```python
from build123d import *

# Parameters (mm, degrees)
SKETCH_1_W           = 23.4
SKETCH_1_H           = 23.4
EXTRUDE_1_DEPTH      = 38
CUT_EXTRUDE_START    = -4.6
SKETCH_1_3_W         = 20.4
SKETCH_1_3_H         = 17
CUT_EXTRUDE_1_DEPTH  = 37.846109588
CUT_EXTRUDE_START_2  = -1
SKETCH_1_4_W         = 10.2
SKETCH_1_4_H         = 10.2
CUT_EXTRUDE_2_DEPTH  = 41.446109588
CHAMFER_2_SIZE       = 3
CUT_EXTRUDE_3_DEPTH  = 47.135127614
CUT_EXTRUDE_4_REACH  = 46.688
CUT_EXTRUDE_5_DEPTH  = 43.900466198
CUT_EXTRUDE_6_DEPTH  = 42.340657953
SKETCH_10_W          = 4
SKETCH_10_H          = 1
CUT_EXTRUDE_10_DEPTH = 12
HOLE_WIZARD_1_D      = 1.8
HOLE_WIZARD_1_DEPTH  = 3.6


with BuildPart() as part:
    # 草图1 → 凸台-拉伸1 (new body)
    with BuildSketch(Plane.XY):
        Rectangle(SKETCH_1_W, SKETCH_1_H)
    extrude(amount=-EXTRUDE_1_DEPTH)

    # 草图1<3> → 切除-拉伸1 (cut, through all)
    with BuildSketch(Plane.XY.offset(CUT_EXTRUDE_START)):
        with Locations((0, 0.8)):
            Rectangle(SKETCH_1_3_W, SKETCH_1_3_H)
    extrude(amount=-CUT_EXTRUDE_1_DEPTH, mode=Mode.SUBTRACT)

    # 草图1<4> → 切除-拉伸2 (cut, through all)
    with BuildSketch(Plane.XY.offset(CUT_EXTRUDE_START_2)):
        Rectangle(SKETCH_1_4_W, SKETCH_1_4_H)
    extrude(amount=-CUT_EXTRUDE_2_DEPTH, mode=Mode.SUBTRACT)

    # 倒角2
    chamfer_2_edges = [part.edges().sort_by_distance(p)[0] for p in [
        (-11.7, 11.7, -19),
        (11.7, 11.7, -19),
    ]]
    chamfer(chamfer_2_edges, length=CHAMFER_2_SIZE)

    # 草图4 → 切除-拉伸3 (cut, through all)
    with BuildSketch(Plane(origin=(11.7, 0, 0), x_dir=(0, 0, -1), z_dir=(1, 0, 0))):
        Polygon((0, -11.7), (38, -11.7), (38, 8.7), (27, 8.7), (27, 5.7), (34, 4), (34, -1), (22, -6.7), (15, -6.7), (15, -8.7), (11.535898385, -8.7), (0, -8.7), align=None)
        Polygon((15, -6.7), (11.535898385, -8.7), (15, -8.7), align=None)
    extrude(amount=-CUT_EXTRUDE_3_DEPTH, mode=Mode.SUBTRACT)

    # 草图5 → 切除-拉伸4 (cut, up to next)
    with BuildSketch(Plane(origin=(0, 11.7, 0), x_dir=(1, 0, 0), z_dir=(0, 1, 0)), mode=Mode.PRIVATE) as cut_extrude_4_sk1:
        Polygon((-11.7, 27), (-8.7, 27), (-3.414837489, 34), (3.585162511, 34), (8.7, 27), (11.7, 27), (11.7, 38), (-11.7, 38), align=None)
    cut_extrude_4_tool1 = extrude(cut_extrude_4_sk1.sketch, amount=-CUT_EXTRUDE_4_REACH, mode=Mode.PRIVATE) & part.part
    add(cut_extrude_4_tool1.solids().sort_by_distance((-10.2, 11.7, -27.258565))[0], mode=Mode.SUBTRACT)

    # 草图6 → 切除-拉伸5 (cut, through all)
    with BuildSketch(Plane(origin=(11.7, 0, 0), x_dir=(0, 0, -1), z_dir=(1, 0, 0))):
        Polygon((29.767949192, 9.3), (31.5, 10.3), (34, 10.3), (34, 9.3), align=None)
    extrude(amount=-CUT_EXTRUDE_5_DEPTH, mode=Mode.SUBTRACT)

    # 草图7 → 切除-拉伸6 (cut, through all)
    with BuildSketch(Plane(origin=(0, 11.7, 0), x_dir=(1, 0, 0), z_dir=(0, 1, 0))):
        Polygon((-11.2, 34), (-10.2, 34), (-10.2, 29.767949192), (-11.2, 31.5), align=None)
        Polygon((10.2, 34), (10.2, 29.767949192), (11.2, 31.5), (11.2, 34), align=None)
    extrude(amount=-CUT_EXTRUDE_6_DEPTH, mode=Mode.SUBTRACT)

    # 草图10 → 切除-拉伸10 (cut)
    with BuildSketch(Plane.XY):
        with Locations((0, 9.8)):
            Rectangle(SKETCH_10_W, SKETCH_10_H)
    extrude(amount=-CUT_EXTRUDE_10_DEPTH, mode=Mode.SUBTRACT)

    # 孔1
    with Locations(Plane(origin=(0, -8.7, 0), x_dir=(-1, 0, 0), z_dir=(0, -1, 0))):
        with Locations((0, 2.3)):
            Hole(HOLE_WIZARD_1_D / 2, depth=HOLE_WIZARD_1_DEPTH)


solid = part.part
```
Input: part model. Units: mm. Frame: model coordinates. A direction names the side the tool comes from. Coordinates: 2 decimals unless noted, no trailing zeros. Loops run counter-clockwise (first coordinate to the right, second up) from the corner with the lowest first, then second, coordinate; pieces in that order, holes last. Notation, with made-up numbers: (84.5, 82.25) - (134.5, 82.25) arc R34 cw to (134.5, 116.25) - close; hole circle Ø2 at (-7, 87). An arc over 180 degrees is marked (long way). Answer in a Markdown table with one row per item.
(1) Material intervals for L1, parallel to Y at x = 0, z = -4.5; L2, parallel to X at y = -2.25, z = -22; L3, parallel to Z at x = 0, y = -6.7, sorted ascending. Write a range as from..to.
Model answer:
| item | result |
|---|---|
| L1 | y = -8.7..-5.1, 5.1..9.3, 10.3..11.7 |
| L2 | x = -11.7..-10.2, 10.2..11.7 |
| L3 | z = -4.6..-3.2, -1.4..0 |
(2) Cut plane D-D on y = 7.25. Output: boundary loops of the cut face in (x, z), plus the area to 3 significant figures.
Model answer:
| item | result |
|---|---|
| outline | (-11.7, -27) - (-10.2, -27) - (-10.2, -4.6) - (10.2, -4.6) - (10.2, -27) - (11.7, -27) - (11.7, 0) - (-11.7, 0) - close |
| area | 175 mm² |
(3) Cut plane A-A on x = 0. Output: boundary loops of the cut face in (y, z), plus the area to 3 significant figures.
Model answer:
| item | result |
|---|---|
| outline | (-8.7, -11.54) - (-7.7, -13.27) - (-7.7, -4.6) - (-5.1, -4.6) - (-5.1, -3.2) - (-8.7, -3.2) - close; (-8.7, -1.4) - (-5.1, -1.4) - (-5.1, -1) - (5.1, -1) - (5.1, -4.6) - (9.3, -4.6) - (9.3, 0) - (-8.7, 0) - close; (9.3, -29.77) - (10.3, -31.5) - (10.3, -34) - (11.7, -34) - (11.7, 0) - (10.3, 0) - (10.3, -12) - (9.3, -12) - close |
| area | 114 mm² |
(4) Set-up query: faces 5 (the face through (0, 2, 0)), 6 (the face through (2, 10, -6)), 7 (the face through (11.2, 1, -33)), 8 (the face through (10.2, 1, -17)), 9 (the face through (-11, -6.7, -19)). Return all of +Z, -Z, +X, -X, +Y, -Y with unobstructed straight access to the full face (end or side cutting, diameter ignored); none if empty.
Model answer:
| item | result |
|---|---|
| face 5 | +Z, +X, -X, +Y, -Y |
| face 6 | +Z |
| face 7 | -Z, +Y, -Y |
| face 8 | -Z |
| face 9 | -Z, +X, -X, -Y |
(5) Pin query (flat end, axial travel): P1, Ø1.2, axis at x = 11, z = -18, coming from the -Y side; P2, Ø0.8, axis at y = 9.5, z = -9, coming from the -X side; P3, Ø0.8, axis at y = 10, z = -4.5, coming from the +X side. Return the tip coordinate at first contact, or that it passes through.
Model answer:
| item | result |
|---|---|
| P1 | stops at y = -6.7 |
| P2 | stops at x = -11.3 |
| P3 | stops at x = 10.8 |
(6) Cut plane B-B on z = -2.3. Output: boundary loops of the cut face in (x, y).
Model answer:
| item | result |
|---|---|
| outline | (-11.7, -8.7) - (-0.9, -8.7) - (-0.9, -5.1) - (-5.1, -5.1) - (-5.1, 5.1) - (5.1, 5.1) - (5.1, -5.1) - (0.9, -5.1) - (0.9, -8.7) - (11.7, -8.7) - (11.7, 8.7) - (8.7, 11.7) - (-8.7, 11.7) - (-11.7, 8.7) - close; hole (-2, 9.3) - (2, 9.3) - (2, 10.3) - (-2, 10.3) - close |
(7) Mould query, pull axis Y, two halves, no side actions, for faces 1 (the face through (-10.2, 1, -17)), 2 (the face through (0, -5.1, -4)), 3 (the face through (11, -6.7, -19)), 4 (the face through (-11.11, 5.05, -29.67)). Classes: pulls with the +Y half, pulls with the -Y half, needs draft (parallel to the pull), parting line crosses it, or undercut.
Model answer:
| item | result |
|---|---|
| face 1 | undercut |
| face 2 | undercut |
| face 3 | pulls with the -Y half |
| face 4 | pulls with the +Y half |
(8) Cut plane C-C on z = -17.5. Output: boundary loops of the cut face in (x, y), plus the area to 3 significant figures.
Model answer:
| item | result |
|---|---|
| outline | (-11.7, -6.7) - (-10.2, -6.7) - (-10.2, 9.3) - (10.2, 9.3) - (10.2, -6.7) - (11.7, -6.7) - (11.7, 8.7) - (8.7, 11.7) - (-8.7, 11.7) - (-11.7, 8.7) - close |
| area | 95.2 mm² |
